Read the model definition and answer for the solid it produces. Units are mm, in the model's axes. Face numbers are marked on the shaded views. A direction names the side the tool comes from. Coordinates: 2 decimals unless noted, no trailing zeros. Loops run counter-clockwise (first coordinate to the right, second up) from the corner with the lowest first, then second, coordinate; pieces in that order, holes last. Notation, with made-up numbers: M 77.25,76 L 116.25,76 A22 ccw 116.25,84 Z; hole C -22,45.5 d11. An arc over 180 degrees is marked long. One line per item, written item: value. Start each with the question number.
```python
from build123d import *

# Parameters (mm, degrees)
F1_DEPTH = 5
F2_D     = 5
F3_SIZE2 = 0.5
F3_SIZE  = 1
F4_W     = 4.25
F4_H     = 26
F5_DEPTH = 1


with BuildPart() as f1:
    # F0 (on Top) → F1 (new body)
    with BuildSketch(Plane.XY):
        with BuildLine():
            Line((60, 0), (0, 0))
            Line((0, 0), (0, -26))
            Line((0, -26), (4.25, -26))
            Line((4.25, -26), (4.25, -13))
            ThreePointArc((4.25, -13), (6.5, -10.75), (8.75, -13))
            Line((8.75, -13), (8.75, -30))
            Line((8.75, -30), (27.5, -30))
            Line((27.5, -30), (27.5, -29))
            ThreePointArc((27.5, -29), (28.0857864376, -27.5857864376), (29.5, -27))
            Line((29.5, -27), (33.5, -27))
            ThreePointArc((33.5, -27), (34.9142135624, -27.5857864376), (35.5, -29))
            Line((35.5, -29), (35.5, -30))
            Line((35.5, -30), (51.25, -30))
            Line((51.25, -30), (51.25, -13))
            ThreePointArc((51.25, -13), (53.5, -10.75), (55.75, -13))
            Line((55.75, -13), (55.75, -26))
            Line((55.75, -26), (60, -26))
            Line((60, -26), (60, 0))
        make_face()
    extrude(amount=-F1_DEPTH)

    # F2 (through all)
    with Locations(Plane.XY):
        with Locations((23, -23)):
            Hole(F2_D / 2)

    # F3
    f3_edges = [f1.edges().sort_by_distance(p)[0] for p in [
        (31.5, -27, -5),
    ]]
    f3_side = f1.faces().sort_by_distance((30.066886, -13.81093, -5))[0]
    chamfer(f3_edges, length=F3_SIZE, length2=F3_SIZE2, reference=f3_side)

    # F4 (on face) → F5 (cut)
    with BuildSketch(Plane(origin=(0, 0, -5), x_dir=(1, 0, 0), z_dir=(0, 0, -1))):
        with Locations((2.125, 13)):
            Rectangle(F4_W, F4_H)
    extrude(amount=-F5_DEPTH, mode=Mode.SUBTRACT)


solid = f1.part
```
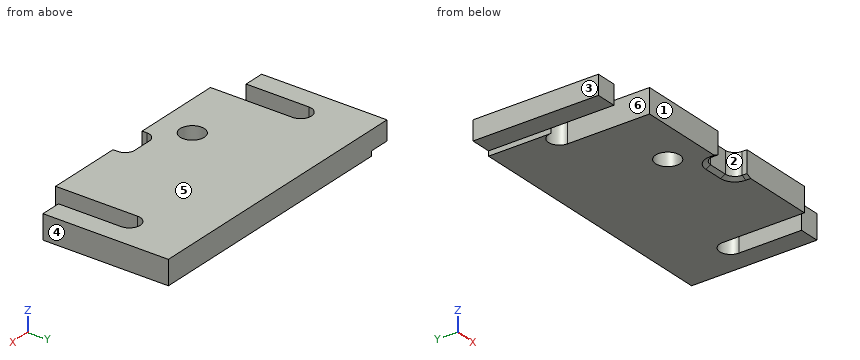
1) Consider line 1 along X through (y, z) = (-13.75, -3.25); line 2 along Y through (x, z) = (23, -3.9); line 3 along Y through (x, z) = (22, -4.7). Determine where each line is inside the solid, lowest interval first.
2) Section B-B (y = -23) is taken. Determine the outline of the cut face in (x, z), then the cut area to 3 significant figures.
3) A tool of negligible diameter and unlimited length cuts with its end or side. For the marked faces 1 and 2, from which of +Z, -Z, +X, -X, +Y, -Y can it reach the whole face along a straight path? Write none if from no direction.
4) Section C-C (x = 23) is taken. Determine the outline of the cut face in (y, z).
5) For a pull along X with two mould halves and no side action, classify the marked faces 3, 4, 5 and 6 as released by +X, released by -X, zero draft, split by the parting line, or undercut.
6) Section D-D (y = -14.25) is taken. Determine the outline of the cut face in (x, z).
7) Flat-ended cylindrical pins translate along their axes: pin 1 (1.2 mm diameter, centred on x = 32, z = -1.5, fed in from -Y); pin 2 (1.1 mm diameter, centred on y = -29.5, z = -2.5, fed in from -X); pin 3 (0.5 mm diameter, centred on y = -29.5, z = -1.5, fed in from +X). Find the tip coordinate at first contact, or state that the pin passes through.
8) Section A-A (z = -2.75) is taken. Determine the outline of the cut face in (x, y).
Results found:
1. line 1: x = 0 to 4.25, 8.75 to 51.25, 55.75 to 60
1. line 2: y = -30 to -25.5, -20.5 to 0
1. line 3: y = -30 to -25.29, -20.71 to 0
2. outline: M 0,-4 L 4.25,-4 L 4.25,0 L 0,0 Z; M 8.75,-5 L 20.5,-5 L 20.5,0 L 8.75,0 Z; M 25.5,-5 L 51.25,-5 L 51.25,0 L 25.5,0 Z; M 55.75,-5 L 60,-5 L 60,0 L 55.75,0 Z
2. area: 226 mm²
3. face 1: +Z, -Z, +X, -X, -Y
3. face 2: +Z, -Z, -Y
4. outline: M -30,-5 L -25.5,-5 L -25.5,0 L -30,0 Z; M -20.5,-5 L 0,-5 L 0,0 L -20.5,0 Z
5. face 3: released by -X
5. face 4: released by +X
5. face 5: zero draft
5. face 6: undercut
6. outline: M 0,-4 L 4.25,-4 L 4.25,0 L 0,0 Z; M 8.75,-5 L 51.25,-5 L 51.25,0 L 8.75,0 Z; M 55.75,-5 L 60,-5 L 60,0 L 55.75,0 Z
7. pin 1: stops at y = -27
7. pin 2: stops at x = 8.75
7. pin 3: stops at x = 51.25
8. outline: M 0,-26 L 4.25,-26 L 4.25,-13 A2.25 cw 8.75,-13 L 8.75,-30 L 27.5,-30 L 27.5,-29 A2 cw 29.5,-27 L 33.5,-27 A2 cw 35.5,-29 L 35.5,-30 L 51.25,-30 L 51.25,-13 A2.25 cw 55.75,-13 L 55.75,-26 L 60,-26 L 60,0 L 0,0 Z; hole C 23,-23 d5
